from build123d import *

# Parameters (mm, degrees)
BOX_W        = 10.5
BOX_H        = 13.2
BOX_DEPTH    = 1.6
SKETCH_R     = 1
SKETCH_R_2   = 2
PAD_DEPTH    = 0.01
SKETCH001_R  = 0.5
POCKET_DEPTH = 1.611
SKETCH002_W  = 2.5
SKETCH002_H  = 2.5
PAD001_DEPTH = 1
FILLET_R     = 0.5
FILLET001_R  = 0.3


with BuildPart() as part:
    # Box → Box (new body)
    with BuildSketch(Plane.XY):
        with Locations((5.25, 6.6)):
            Rectangle(BOX_W, BOX_H)
    extrude(amount=BOX_DEPTH)

    # Sketch → Pad (new body)
    with BuildSketch(Plane.XY.offset(1.6)):
        with Locations((1.44, 1.5)):
            Circle(SKETCH_R)
        with Locations((3.98, 1.5)):
            Circle(SKETCH_R)
        with Locations((6.52, 1.5)):
            Circle(SKETCH_R)
        with Locations((9.06, 1.5)):
            Circle(SKETCH_R)
        with Locations((7.75, 10.5)):
            Circle(SKETCH_R_2)
    extrude(amount=PAD_DEPTH)

    # Sketch001 → Pocket (cut, through all)
    with BuildSketch(Plane.XY.offset(1.61)):
        with Locations((1.44, 1.5)):
            Circle(SKETCH001_R)
        with Locations((3.98, 1.5)):
            Circle(SKETCH001_R)
        with Locations((6.52, 1.5)):
            Circle(SKETCH001_R)
        with Locations((9.06, 1.5)):
            Circle(SKETCH001_R)
        with BuildLine():
            ThreePointArc((6.25, 10.5), (6.68934, 9.43934), (7.75, 9))
            Line((7.75, 9), (10.5, 9))
            Line((10.5, 9), (10.5, 13.2))
            Line((6.25, 13.2), (10.5, 13.2))
            Line((6.25, 10.5), (6.25, 13.2))
        make_face()
    extrude(amount=-POCKET_DEPTH, mode=Mode.SUBTRACT)

    # Sketch002 → Pad001 (new body)
    with BuildSketch(Plane(origin=(0, 0, 0), x_dir=(1, 0, 0), z_dir=(0, 0, -1))):
        with Locations((2.95, -10.6)):
            Rectangle(SKETCH002_W, SKETCH002_H)
    extrude(amount=PAD001_DEPTH)

    # Fillet
    fillet_edges = [part.edges().sort_by_distance(p)[0] for p in [
        (1.7, 11.85, -0.5),
        (4.2, 11.85, -0.5),
        (4.2, 9.35, -0.5),
        (1.7, 9.35, -0.5),
    ]]
    fillet(fillet_edges, radius=FILLET_R)

    # Fillet001
    fillet001_edges = [part.edges().sort_by_distance(p)[0] for p in [
        (4.2, 10.6, -1),
        (2.95, 9.35, -1),
        (1.7, 10.6, -1),
        (2.95, 11.85, -1),
    ]]
    fillet(fillet001_edges, radius=FILLET001_R)


solid = part.part
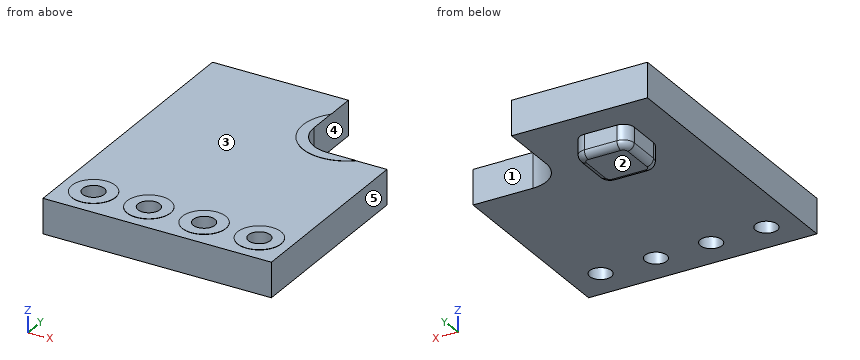
Build history of the part. All positions in model axes, mm. Face numbers are marked on the shaded views. A direction names the side the tool comes from. Round coordinates to 2 decimals unless told otherwise and drop trailing zeros. Write each loop counter-clockwise with the first axis right and the second up, starting at its lowest first coordinate (ties: lowest second). Pieces come first, ordered by that corner, then holes. Notation, with made-up numbers: M -26.75,67.5 L -15.75,67.5 A26 cw -15.75,98.5 Z; hole C 39.5,70.5 d4. An arc over 180 degrees is marked long. Answer in a Markdown table with one row per item.
1. Probe L1, parallel to Y at x = 1.44, z = 1.1; L2, parallel to X at y = 11.25, z = 1.45; L3, parallel to Z at x = 0.5, y = 8.75. List the from-to ranges inside material, lowest first. Write a range as [from, to].
Geometry check:
| item | result |
|---|---|
| L1 | [0, 1], [2, 13.2] |
| L2 | [0, 6.25] |
| L3 | [0, 1.6] |
2. Saw through at B-B (z = 1.2). List the corners of the cut face in (x, y).
Geometry check:
| item | result |
|---|---|
| outline | M 0,0 L 10.5,0 L 10.5,9 L 7.75,9 A1.5 cw 6.25,10.5 L 6.25,13.2 L 0,13.2 Z; hole C 1.44,1.5 d1; hole C 3.98,1.5 d1; hole C 6.52,1.5 d1; hole C 9.06,1.5 d1 |
3. Flat gauge pins, fed straight in: P1, Ø1, axis at x = 6.5, y = 7, coming from the +Z side; P2, Ø0.6, axis at y = 10.5, z = -0.5, coming from the +X side; P3, Ø1, axis at y = 10, z = 0, coming from the +X side. Where does each tip first touch, or does it go through?
Geometry check:
| item | result |
|---|---|
| P1 | z = 1.6 |
| P2 | x = 4.2 |
| P3 | x = 6.63 |
4. Which spindle directions (+Z, -Z, +X, -X, +Y, -Y) get a long thin tool onto all of the face, cutting with end or side? Do the marked faces 4 and 5. Say none if no direction does.
Geometry check:
| item | result |
|---|---|
| face 4 | +Z, -Z, +X, +Y |
| face 5 | +Z, -Z, +X, +Y, -Y |
5. Mould opens along Z. For the marked faces 1, 2 and 3 say: +Z half, -Z half, draft (parallel to the pull), parting line (faces both ways), or undercut.
Geometry check:
| item | result |
|---|---|
| face 1 | draft |
| face 2 | -Z half |
| face 3 | +Z half |
6. Saw through at C-C (y = 1.5). State how many separate pieces and enclosed holes the cut face has, and give its area (3 significant figures).
Geometry check:
| item | result |
|---|---|
| separate pieces | 5 |
| enclosed holes | 0 |
| area | 10.4 mm2 |
